Design review of the part built by this model. Coordinates are the model's own, in mm. A direction names the side the tool comes from. Give positions to 0.01 mm unless a question says otherwise; leave off trailing zeros. Order: outer loops, then holes, each group sorted by start corner. A loop starts at its lowest first (then second) coordinate and runs counter-clockwise, first axis right, second up. Notation, with made-up numbers: (28.5, 14) -> (41.5, 14) arc R24 ccw to (41.5, 35) -> close; hole circle Ø7 at (32.25, 49.5). An arc over 180 degrees is marked (long way). One line per item, written item: value.
from build123d import *

# Parameters (mm, degrees)
SKETCH1_R           = 13.5
SKETCH1_R_2         = 10
BOSS_EXTRUDE1_DEPTH = 2
CUT_EXTRUDE1_START  = 2
SKETCH2_R           = 12.5
SKETCH2_R_2         = 11
CUT_EXTRUDE1_DEPTH  = 0.2
CUT_EXTRUDE2_START  = -1.8
SKETCH2_2_R         = 12.5
SKETCH2_2_R_2       = 11
CUT_EXTRUDE2_DEPTH  = 0.2


with BuildPart() as part:
    # Sketch1 → Boss-Extrude1 (new, symmetric)
    with BuildSketch(Plane(origin=(0, 0, 0), x_dir=(1, 0, 0), z_dir=(0, 1, 0))):
        with Locations(Location((0, 0, 0), (0, 0, 270))):
            Circle(SKETCH1_R)
        with Locations(Location((0, 0, 0), (0, 0, 270))):
            Circle(SKETCH1_R_2, mode=Mode.SUBTRACT)
    extrude(amount=BOSS_EXTRUDE1_DEPTH, both=True)

    # Sketch2 → Cut-Extrude1 (cut)
    with BuildSketch(Plane.XZ.offset(CUT_EXTRUDE1_START)):
        with Locations(Location((0, 0, 0), (0, 0, 90))):
            Circle(SKETCH2_R)
        with Locations(Location((0, 0, 0), (0, 0, 90))):
            Circle(SKETCH2_R_2, mode=Mode.SUBTRACT)
    extrude(amount=-CUT_EXTRUDE1_DEPTH, mode=Mode.SUBTRACT)

    # Sketch2<2> → Cut-Extrude2 (cut)
    with BuildSketch(Plane.XZ.offset(CUT_EXTRUDE2_START)):
        with Locations(Location((0, 0, 0), (0, 0, 90))):
            Circle(SKETCH2_2_R)
        with Locations(Location((0, 0, 0), (0, 0, 90))):
            Circle(SKETCH2_2_R_2, mode=Mode.SUBTRACT)
    extrude(amount=-CUT_EXTRUDE2_DEPTH, mode=Mode.SUBTRACT)


solid = part.part
Item 1: To check wall thickness, follow line 1 along X through (y, z) = (1.95, 0); line 2 along Y through (x, z) = (11.25, 1.25); line 3 along X through (y, z) = (0.8, 0). State the ranges of each line that lie inside material, in increasing order. Write a range as from..to.
Returned:
line 1: -13.5..-12.5, -11..-10, 10..11, 12.5..13.5
line 2: -1.8..1.8
line 3: -13.5..-10, 10..13.5
Item 2: Machinability: for faces 4 (the flat face through (10, 1.8, 5)), 5 (the cylindrical face through (-9.76, -0.03, -2.17)), which of the approach directions +Z, -Z, +X, -X, +Y, -Y give a long, thin tool a straight path to every point of the face, cutting with its end or side? Answer none if there is none.
Returned:
face 4: +Y
face 5: +Y, -Y
Item 3: Add section A-A on x = 0. Give the boundary of the cut face in (y, z).
Returned:
outline: (-2, -13.5) -> (2, -13.5) -> (2, -12.5) -> (1.8, -12.5) -> (1.8, -11) -> (2, -11) -> (2, -10) -> (-2, -10) -> (-2, -11) -> (-1.8, -11) -> (-1.8, -12.5) -> (-2, -12.5) -> close; (-2, 10) -> (2, 10) -> (2, 11) -> (1.8, 11) -> (1.8, 12.5) -> (2, 12.5) -> (2, 13.5) -> (-2, 13.5) -> (-2, 12.5) -> (-1.8, 12.5) -> (-1.8, 11) -> (-2, 11) -> close
Item 4: Draft analysis for pull direction Z (two halves, no side actions). For faces 1 (the flat face through (-9, 2, 9)), 2 (the flat face through (10, -1.8, 5)), 3 (the cylindrical face through (-13.18, 0.03, -2.93)), state which applies: pulls with the +Z half, pulls with the -Z half, needs draft (parallel to the pull), parting line crosses it, or undercut.
Returned:
face 1: needs draft
face 2: undercut
face 3: parting line crosses it
Item 5: Add section B-B on z = 0. Give the boundary of the cut face in (x, y).
Returned:
outline: (-13.5, -2) -> (-12.5, -2) -> (-12.5, -1.8) -> (-11, -1.8) -> (-11, -2) -> (-10, -2) -> (-10, 2) -> (-11, 2) -> (-11, 1.8) -> (-12.5, 1.8) -> (-12.5, 2) -> (-13.5, 2) -> close; (10, -2) -> (11, -2) -> (11, -1.8) -> (12.5, -1.8) -> (12.5, -2) -> (13.5, -2) -> (13.5, 2) -> (12.5, 2) -> (12.5, 1.8) -> (11, 1.8) -> (11, 2) -> (10, 2) -> close
Item 6: Clearance check with a flat-ended pin moving along its axis: P1, Ø1, axis at y = 0.5, z = -2.5, coming from the +X side. State where the tip first meets the part, or that it passes through.
Returned:
P1: x = 13.35
Item 7: Add section C-C on y = -1.45. Give the boundary of the cut face in (x, z), plus the area to 3 significant figures.
Returned:
outline: circle Ø27 at (0, 0); hole circle Ø20 at (0, 0)
area: 258 mm²
